The listing builds one solid part. Answer for the finished solid, in the listing's coordinates (mm). Face numbers are marked on the shaded views. A direction names the side the tool comes from. Round coordinates to 2 decimals unless told otherwise and drop trailing zeros. Write each loop counter-clockwise with the first axis right and the second up, starting at its lowest first coordinate (ties: lowest second). Pieces come first, ordered by that corner, then holes.
Item 1: Find section A-A on y = 3.5. Give the vertices of the cut face in (x, z), then the cut area to 3 significant figures.
Item 2: Find section D-D on x = -12. Give the vertices of the cut face in (y, z), then the cut area to 3 significant figures.
Item 3: A tool of negligible diameter and unlimited length cuts with its end or side. For the marked faces 1 and 2, from which of +Z, -Z, +X, -X, +Y, -Y can it reach the whole face along a straight path? Write none if from no direction.
Item 4: Find the intervals of material crossed by probe 1 along Y at (x, z) = (10, -11); probe 2 along Y at (x, z) = (-1.5, -3); probe 3 along X at (y, z) = (4.3, 0), in increasing order.
Item 5: Each of these flat-tipped pins is pushed along its axis until it touches: pin 1 (1.7 mm diameter, centred on y = 3, z = -16.5, fed in from -X); pin 2 (3 mm diameter, centred on x = -9, z = 3.5, fed in from +Y); pin 3 (0.5 mm diameter, centred on x = -0.5, z = 16, fed in from +Y). Where does it stop, or does it pass through?
Item 6: Find section C-C on y = 0.75. Give the number of separate pieces and of enclosed holes in the cut face, then the cut area to 3 significant figures.
Item 7: For a pull along X with two mould halves and no side action, classify the marked faces 3, 4, 5 and 6 as +X half, -X half, draft (parallel to the pull), parting line (faces both ways), or undercut.
Item 8: Find section B-B on x = 8. Give the vertices of the cut face in (y, z).
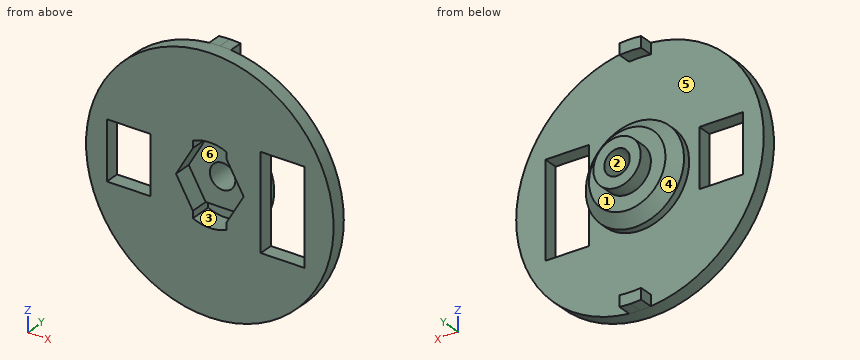
```python
from build123d import *

# Parameters (mm, degrees)
SKETCH1_R           = 17
SKETCH1_R_2         = 15.5
SKETCH1_R_3         = 6.75
SKETCH1_W           = 6
SKETCH1_H           = 8
SKETCH1_H_2         = 13
SKETCH1_R_4         = 3.25
SKETCH1_R_5         = 1.75
BOSS_EXTRUDE1_DEPTH = 2
SKETCH1_3_R         = 6.75
SKETCH1_3_R_2       = 1.75
BOSS_EXTRUDE2_DEPTH = 4.5
SKETCH1_4_R         = 3.25
SKETCH1_4_R_2       = 1.75
BOSS_EXTRUDE3_DEPTH = 6.5
SKETCH1_5_R         = 3.25
SKETCH1_5_R_2       = 1.75
CUT_EXTRUDE1_DEPTH  = 2.5
BOSS_EXTRUDE4_DEPTH = 1.9
CUT_EXTRUDE2_DEPTH  = 3
CHAMFER1_SIZE       = 1.5


with BuildPart() as part:
    # Sketch1 → Boss-Extrude1 (new body)
    # profile 1 of 5: a face of its own
    with BuildSketch(Plane(origin=(0, 0, 0), x_dir=(1, 0, 0), z_dir=(0, 1, 0))):
        with Locations(Location((0, 0, 0), (0, 0, 270))):
            Circle(SKETCH1_R)
        Circle(SKETCH1_R_2, mode=Mode.SUBTRACT)
    # profile 2 of 5: a face of its own
    with BuildSketch(Plane(origin=(0, 0, 0), x_dir=(1, 0, 0), z_dir=(0, 1, 0))):
        Circle(SKETCH1_R_2)
        Circle(SKETCH1_R_3, mode=Mode.SUBTRACT)
        with Locations((-11.142, 0)):
            Rectangle(SKETCH1_W, SKETCH1_H, mode=Mode.SUBTRACT)
        with Locations((9.99, 0)):
            Rectangle(SKETCH1_W, SKETCH1_H_2, mode=Mode.SUBTRACT)
    # profile 3 of 5: a face of its own
    with BuildSketch(Plane(origin=(0, 0, 0), x_dir=(1, 0, 0), z_dir=(0, 1, 0))):
        Circle(SKETCH1_R_3)
        Polygon((2.323834833, -4.025), (4.647669667, 0), (2.323834833, 4.025), (-2.323834833, 4.025), (-4.647669667, 0), (-2.323834833, -4.025), align=None, mode=Mode.SUBTRACT)
    # profile 4 of 5: a face of its own
    with BuildSketch(Plane(origin=(0, 0, 0), x_dir=(1, 0, 0), z_dir=(0, 1, 0))):
        Polygon((-2.323834833, -4.025), (2.323834833, -4.025), (4.647669667, 0), (2.323834833, 4.025), (-2.323834833, 4.025), (-4.647669667, 0), align=None)
        Circle(SKETCH1_R_4, mode=Mode.SUBTRACT)
    # profile 5 of 5: a face of its own
    with BuildSketch(Plane(origin=(0, 0, 0), x_dir=(1, 0, 0), z_dir=(0, 1, 0))):
        Circle(SKETCH1_R_4)
        with Locations(Location((0, 0, 0), (0, 0, 270))):
            Circle(SKETCH1_R_5, mode=Mode.SUBTRACT)
    extrude(amount=BOSS_EXTRUDE1_DEPTH)

    # Sketch1_3 → Boss-Extrude2 (add)
    with BuildSketch(Plane(origin=(0, 0, 0), x_dir=(1, 0, 0), z_dir=(0, 1, 0))):
        with Locations(Location((0, 0, 0), (0, 0, 270))):
            Circle(SKETCH1_3_R)
        with Locations(Location((0, 0, 0), (0, 0, 270))):
            Circle(SKETCH1_3_R_2, mode=Mode.SUBTRACT)
    extrude(amount=BOSS_EXTRUDE2_DEPTH)

    # Sketch1_4 → Boss-Extrude3 (add)
    with BuildSketch(Plane(origin=(0, 0, 0), x_dir=(1, 0, 0), z_dir=(0, 1, 0))):
        with Locations(Location((0, 0, 0), (0, 0, 90))):
            Circle(SKETCH1_4_R)
        with Locations(Location((0, 0, 0), (0, 0, 270))):
            Circle(SKETCH1_4_R_2, mode=Mode.SUBTRACT)
    extrude(amount=BOSS_EXTRUDE3_DEPTH)

    # Sketch1_5 → Cut-Extrude1 (cut)
    # profile 1 of 2: a face of its own
    with BuildSketch(Plane(origin=(0, 0, 0), x_dir=(1, 0, 0), z_dir=(0, 1, 0))):
        Polygon((-2.323834833, -4.025), (2.323834833, -4.025), (4.647669667, 0), (2.323834833, 4.025), (-2.323834833, 4.025), (-4.647669667, 0), align=None)
        with Locations(Location((0, 0, 0), (0, 0, 90))):
            Circle(SKETCH1_5_R, mode=Mode.SUBTRACT)
    # profile 2 of 2: a face of its own
    with BuildSketch(Plane(origin=(0, 0, 0), x_dir=(1, 0, 0), z_dir=(0, 1, 0))):
        with Locations(Location((0, 0, 0), (0, 0, 90))):
            Circle(SKETCH1_5_R)
        with Locations(Location((0, 0, 0), (0, 0, 270))):
            Circle(SKETCH1_5_R_2, mode=Mode.SUBTRACT)
    extrude(amount=CUT_EXTRUDE1_DEPTH, mode=Mode.SUBTRACT)

    # Sketch2 → Boss-Extrude4 (add)
    with BuildSketch(Plane(origin=(0, 2, 0), x_dir=(1, 0, 0), z_dir=(0, 1, 0))):
        with BuildLine():
            ThreePointArc((7e-09, 17), (-0.745717799, 16.983636388), (-1.49, 16.934577054))
            Line((-1.49, 16.934577054), (-1.49, 15.428217655))
            ThreePointArc((-1.49, 15.428217655), (0, 15.5), (1.49, 15.428217655))
            Line((1.49, 15.428217655), (1.49, 16.934577054))
            ThreePointArc((1.49, 16.934577054), (0.745717806, 16.983636388), (7e-09, 17))
        make_face()
        with BuildLine():
            Line((-1.49, -15.428217655), (-1.49, -16.934577054))
            ThreePointArc((-1.49, -16.934577054), (-0.745717806, -16.983636388), (-7e-09, -17))
            ThreePointArc((-7e-09, -17), (0.745717799, -16.983636388), (1.49, -16.934577054))
            Line((1.49, -16.934577054), (1.49, -15.428217655))
            ThreePointArc((1.49, -15.428217655), (0, -15.5), (-1.49, -15.428217655))
        make_face()
    extrude(amount=BOSS_EXTRUDE4_DEPTH)

    # Sketch4 → Cut-Extrude2 (cut)
    with BuildSketch(Plane.XZ):
        with BuildLine():
            Line((-2.323834833, 4.025), (2.323666704, 4.025))
            Line((2.323666704, 4.025), (2.323666704, 4.98503491))
            ThreePointArc((2.323666704, 4.98503491), (-9.275e-05, 5.499999999), (-2.323834833, 4.984956536))
            Line((-2.323834833, 4.984956536), (-2.323834833, 4.025))
        make_face()
        with BuildLine():
            Line((2.323666704, -4.025), (2.323666704, -4.98503491))
            ThreePointArc((2.323666704, -4.98503491), (0, -5.5), (-2.323666704, -4.98503491))
            Line((-2.323666704, -4.98503491), (-2.323834833, -4.025))
            Line((-2.323834833, -4.025), (2.323666704, -4.025))
        make_face()
    extrude(amount=-CUT_EXTRUDE2_DEPTH, mode=Mode.SUBTRACT)

    # Chamfer1
    chamfer1_edges = [part.edges().sort_by_distance(p)[0] for p in [
        (0, 4.5, -6.75),
    ]]
    chamfer(chamfer1_edges, length=CHAMFER1_SIZE)


solid = part.part
```
Check values:
1. outline: circle Ø12.5 at (0, 0); (-1.49, -16.93) arc R17 ccw to (1.49, -16.93) - (1.49, -15.43) arc R15.5 cw to (-1.49, -15.43) - close; (-1.49, 15.43) arc R15.5 cw to (1.49, 15.43) - (1.49, 16.93) arc R17 ccw to (-1.49, 16.93) - close; hole circle Ø3.5 at (0, 0)
1. area: 122 mm2
2. outline: (0, -12.04) - (2, -12.04) - (2, -4) - (0, -4) - close; (0, 4) - (2, 4) - (2, 12.04) - (0, 12.04) - close
2. area: 32.2 mm2
3. face 1: +Y
3. face 2: +Y, -Y
4. probe 1: y = 0 to 2
4. probe 2: y = 2.5 to 4.5
4. probe 3: x = -5.45 to -1.75, 1.75 to 5.45
5. pin 1: stops at x = -1.49
5. pin 2: stops at y = 2
5. pin 3: stops at y = 3.9
6. separate pieces: 1
6. enclosed holes: 3
6. area: 714 mm2
7. face 3: undercut
7. face 4: parting line
7. face 5: draft
7. face 6: undercut
8. outline: (0, -15) - (2, -15) - (2, -6.5) - (0, -6.5) - close; (0, 6.5) - (2, 6.5) - (2, 15) - (0, 15) - close
